Geometry: final body of the model. Coordinates: model frame, mm. A direction names the side the tool comes from. Give positions to 0.01 mm unless a question says otherwise; leave off trailing zeros. Write each loop counter-clockwise with the first axis right and the second up, starting at its lowest first coordinate (ties: lowest second). Pieces come first, ordered by that corner, then holes. Notation, with made-up numbers: M 28.25,4.5 L 86.25,4.5 A22 ccw 86.25,21.5 Z; hole C 20.25,1 d2. An arc over 180 degrees is marked long. Use a Markdown table: item, result. Add a question column.
1) Section B-B on z = -14. Return the cut outline in (x, y), then the cut area to 3 significant figures.
2) Line query: line 1 (X direction, y = 55, z = 10.5); line 2 (Z direction, x = 1.75, y = 56.5); line 3 (Z direction, x = -4.25, y = 103.5). Output: solid intervals per line, ascending.
3) Set-up query: faces 4 (the flat face through (0, 60, 24)), 5 (the flat face through (0, 59, -24)), 6 (the flat face through (-7.15, 10, -2.2)), 7 (the flat face through (5, 60, 0)), 8 (the flat face through (0, 4, 30)). Return all of +Z, -Z, +X, -X, +Y, -Y with unobstructed straight access to the full face (end or side cutting, diameter ignored); none if empty.
4) Draft query along Z for faces 1 (the flat face through (10, 4, 0)), 2 (the cylindrical face through (0, 100, 0)), 3 (the cylindrical face through (-0.1, 10.57, -24.6)). Return one class per face: +Z half, -Z half, draft (parallel to the pull), parting line (faces both ways), or undercut.
5) Section C-C on y = 25. Return the cut outline in (x, z), then the cut area to 3 significant figures.
6) Pin query (flat end, axial travel): pin 1 (3 mm diameter, centred on y = 75.5, z = -4.5, fed in from +X); pin 2 (6 mm diameter, centred on x = 5, z = -16, fed in from +Y); pin 3 (10 mm diameter, centred on x = 1, y = 16.5, fed in from -Z). Return the tip coordinate at first contact, or that it passes through.
7) Section A-A on x = 3. Return the cut outline in (y, z).
```python
from build123d import *

# Parameters (mm, degrees)
SKETCH_1_W      = 20
SKETCH_1_H      = 60
EXTRUDE_1_DEPTH = 10
EXTRUDE_3_DEPTH = 5
FILLET_1_R      = 2


with BuildPart() as part:
    # 스케치1 → 보스-돌출1 (new body)
    with BuildSketch(Plane(origin=(0, 0, 0), x_dir=(1, 0, 0), z_dir=(0, 1, 0))):
        Rectangle(SKETCH_1_W, SKETCH_1_H)
    extrude(amount=EXTRUDE_1_DEPTH)

    # 스케치5 → 보스-돌출3 (add, symmetric)
    with BuildSketch(Plane(origin=(0, 0, 0), x_dir=(0, 0, -1), z_dir=(1, 0, 0))):
        with BuildLine():
            Line((-24, 0), (24, 0))
            Line((24, 0), (24, 100))
            Line((24, 100), (24, 106.934267379))
            ThreePointArc((24, 106.934267379), (0, 100), (-24, 106.934267379))
            Line((-24, 106.934267379), (-24, 100))
            Line((-24, 100), (-24, 0))
        make_face()
    extrude(amount=EXTRUDE_3_DEPTH, both=True)

    # 필렛1
    fillet_1_edges = [part.edges().sort_by_distance(p)[0] for p in [
        (10, 10, 0),
        (0, 10, -30),
        (0, 10, -24),
        (0, 10, 24),
        (-5, 10, 0),
        (5, 10, 0),
        (-10, 10, 0),
        (-10, 5, -30),
        (10, 5, -30),
        (10, 5, 30),
        (-10, 5, 30),
        (0, 10, 30),
    ]]
    fillet(fillet_1_edges, radius=FILLET_1_R)


solid = part.part
```
Found:
| question | item | result |
|---|---|---|
| 1 | outline | M -10,0 L 10,0 L 10,8 A2 ccw 8,10 L 7,10 A2 cw 5,12 L 5,102.23 L -5,102.23 L -5,12 A2 cw -7,10 L -8,10 A2 ccw -10,8 Z |
| 1 | area | 1,120 mm² |
| 2 | line 1 | -5 to 5 |
| 2 | line 2 | -24 to 24 |
| 2 | line 3 | -24 to -17.4, 17.4 to 24 |
| 3 | face 4 | +Z, +X, -X, +Y |
| 3 | face 5 | -Z, +X, -X, +Y |
| 3 | face 6 | +Y |
| 3 | face 7 | +Z, -Z, +X, +Y |
| 3 | face 8 | +Z, +X, -X, +Y, -Y |
| 4 | face 1 | draft |
| 4 | face 2 | undercut |
| 4 | face 3 | -Z half |
| 5 | outline | M -5,-24 L 5,-24 L 5,24 L -5,24 Z |
| 5 | area | 480 mm² |
| 6 | pin 1 | x = 5 |
| 6 | pin 2 | y = 104.21 |
| 6 | pin 3 | z = -24.06 |
| 7 | outline | M 0,-30 L 8,-30 A2 ccw 10,-28 L 10,-26 A2 cw 12,-24 L 106.93,-24 A45 cw 106.93,24 L 12,24 A2 cw 10,26 L 10,28 A2 ccw 8,30 L 0,30 Z |
